Autodesk Fusion 360 part; units mm, degrees
sketch "草图1" plane through (0, 0, 0) normal (0, 1, 0) x (1, 0, 0)
  circle A0 centre (0, 0) radius 46.5
  circle A1 centre (0, 0) radius 47.5
  circle A2 centre (0, 0) radius 33.5
  circle A3 centre (0, 0) radius 34.5
  circle A4 centre (0, 0) radius 45.5
  circle A5 centre (0, 0) radius 30
  circle A6 centre (0, 0) radius 29
  circle A7 centre (0, 0) radius 31
  dimension "d1" = 93
  dimension "d2" = 95
  dimension "d5" = 67
  dimension "d6" = 69
  dimension "d21" = 91
  dimension "d26" = 60
  dimension "d29" = 58
  dimension "d30" = 62
extrude "拉伸8" add sketch "草图1" along normal blind 60 draft 12.3 contours A3
extrude "拉伸9" cut sketch "草图1" along normal blind 60 draft 12.3 contours A2 | A5 | A6 | A7
extrude "拉伸11" add sketch "草图1" against normal blind 30 contours A3
sketch "草图5" plane through (0, -30, 0) normal (0, -1, 0) x (1, 0, 0)
  circle A0 centre (0, 0) radius 33.5
  circle A1 centre (0, 0) radius 34.5
extrude "拉伸13" add sketch "草图5" along normal blind 100 draft 20
extrude "拉伸14" cut sketch "草图5" along normal blind 100 draft 20 contours A0
sketch "草图6" plane through (0, -130, 0) normal (0, -1, 0) x (1, 0, 0)
  circle A0 centre (0, 0) radius 69.897
  circle A1 centre (0, 0) radius 70.897
extrude "拉伸15" add sketch "草图6" against normal blind 2 draft -20 contours A0
Build history of the part. All positions in model axes, mm. A direction names the side the tool comes from. Round coordinates to 2 decimals unless told otherwise and drop trailing zeros. Order: outer loops, then holes, each group sorted by start corner. A loop starts at its lowest first (then second) coordinate and runs counter-clockwise, first axis right, second up. Notation, with made-up numbers: (-4, -25.75) -> (21, -25.75) arc R6 cw to (21, -18.75) -> close; hole circle Ø5 at (79, 0.25). An arc over 180 degrees is marked (long way). Answer in a Markdown table with one row per item.
1) Which spindle directions (+Z, -Z, +X, -X, +Y, -Y) get a long thin tool onto all of the face, cutting with end or side? Do faces 4 (the flat face through (35, 60, 31)), 5 (the flat face through (-1, -128, 1)), 6 (the cylindrical face through (-7.262, -14.79, 32.703)). Say none if no direction does.
Values:
| item | result |
|---|---|
| face 4 | +Z, -Z, +X, -X, +Y |
| face 5 | none |
| face 6 | +Y |
2) Mould opens along X. For faces 1 (the conical face through (-35.603, -58.478, -27.3)), 2 (the conical face through (36.89, 23.75, -11.62)), 3 (the flat face through (-1, -130, 1)) say: released by +X, released by -X, zero draft, split by the parting line, or undercut.
Values:
| item | result |
|---|---|
| face 1 | split by the parting line |
| face 2 | undercut |
| face 3 | zero draft |
3) Band-saw the part on C-C on z = 0. Give the cut face in (x, y).
Values:
| item | result |
|---|---|
| outline | (-70.9, -130) -> (70.9, -130) -> (34.5, -30) -> (34.5, 0) -> (47.58, 60) -> (46.58, 60) -> (33.5, 0) -> (33.5, -30) -> (69.17, -128) -> (-69.17, -128) -> (-33.5, -30) -> (-33.5, 0) -> (-46.58, 60) -> (-47.58, 60) -> (-34.5, 0) -> (-34.5, -30) -> close |
4) Pin check, flat tips, straight feed: P1, Ø5, axis at x = 30.5, y = -69, coming from the +Z side; P2, Ø12, axis at x = 10, y = -25.5, coming from the +Z side; P3, Ø12, axis at y = 14, z = 34.5, coming from the -X side. Stop position of each tip, or through.
Values:
| item | result |
|---|---|
| P1 | z = 40.16 |
| P2 | z = 34.27 |
| P3 | x = -24.74 |
5) Band-saw the part on D-D on y = 43. Give the cut face in (x, z).
Values:
| item | result |
|---|---|
| outline | circle Ø87.75 at (0, 0); hole circle Ø85.75 at (0, 0) |
6) Wall check: L1, parallel to X at y = -19.75, z = 0; L2, parallel to Y at x = -22.5, z = 18. Give the ranges that are in metal, low to high.
Values:
| item | result |
|---|---|
| L1 | -34.5 to -33.5, 33.5 to 34.5 |
| L2 | -130 to -128 |
7) Band-saw the part on A-A on x = 0. Give the cut face in (y, z), and give its area (3 significant figures).
Values:
| item | result |
|---|---|
| outline | (-130, -70.9) -> (-30, -34.5) -> (0, -34.5) -> (60, -47.58) -> (60, -46.58) -> (0, -33.5) -> (-30, -33.5) -> (-128, -69.17) -> (-128, 69.17) -> (-30, 33.5) -> (0, 33.5) -> (60, 46.58) -> (60, 47.58) -> (0, 34.5) -> (-30, 34.5) -> (-130, 70.9) -> close |
| area | 658 mm2 |
8) Band-saw the part on B-B on y = -107. Give the cut face in (x, z), and give its area (3 significant figures).
Values:
| item | result |
|---|---|
| outline | circle Ø125.05 at (0, 0); hole circle Ø123.05 at (0, 0) |
| area | 390 mm2 |
